from build123d import *

# Parameters (mm, degrees)
SKETCH_W        = 36
SKETCH_H        = 29
SKETCH_R        = 11
PAD_DEPTH       = 7
SKETCH001_R     = 2.5
POCKET_DEPTH    = 29.001
CHAMFER_SIZE    = 1
CHAMFER001_SIZE = 1
CHAMFER002_SIZE = 1


with BuildPart() as part:
    # Sketch → Pad (new body)
    with BuildSketch(Plane.XY):
        Rectangle(SKETCH_W, SKETCH_H)
        Circle(SKETCH_R, mode=Mode.SUBTRACT)
    extrude(amount=PAD_DEPTH)

    # Sketch001 (on Face3 of Pad) → Pocket (cut, through all)
    with BuildSketch(Plane.XZ.offset(14.5)):
        with Locations((13.5, 3.5)):
            Circle(SKETCH001_R)
        with Locations((-13.5, 3.5)):
            Circle(SKETCH001_R)
    extrude(amount=-POCKET_DEPTH, mode=Mode.SUBTRACT)

    # Chamfer
    chamfer_edges = [part.edges().sort_by_distance(p)[0] for p in [
        (18, -14.5, 3.5),
    ]]
    chamfer(chamfer_edges, length=CHAMFER_SIZE)

    # Chamfer001
    chamfer001_edges = [part.edges().sort_by_distance(p)[0] for p in [
        (-18, -14.5, 3.5),
    ]]
    chamfer(chamfer001_edges, length=CHAMFER001_SIZE)

    # Chamfer002
    chamfer002_edges = [part.edges().sort_by_distance(p)[0] for p in [
        (18, 14.5, 3.5),
        (-18, 14.5, 3.5),
    ]]
    chamfer(chamfer002_edges, length=CHAMFER002_SIZE)


solid = part.part
Could you check a few things on this model? Use its own coordinates, in mm. Round coordinates to 2 decimals unless told otherwise and drop trailing zeros. Write each loop counter-clockwise with the first axis right and the second up, starting at its lowest first coordinate (ties: lowest second). Pieces come first, ordered by that corner, then holes. Notation, with made-up numbers: (67.5, 76.5) - (102.5, 76.5) arc R13 ccw to (102.5, 87.5) - close; hole circle Ø2 at (35.25, 32). An arc over 180 degrees is marked (long way). Put each result on its own line as item: value. Start each with the question number.
(1) Thinking about a two-plate mould opening in Z: for faces 1 (the flat face through (-12, 0, 7)), 2 (the cylindrical face through (-16, -0.2, 3.6)), 3 (the flat face through (17.5, 14, 3.5)), 4 (the cylindrical face through (11.66, -0.2, 5.19)), which applies, released by +Z, released by -Z, zero draft, split by the parting line, or undercut?
(2) I want a section at D-D, the plane y = -1.5. Please give me the cut outline in (x, z), plus the area to 3 significant figures.
(3) I want a section at B-B, the plane z = 3.5. Please give me the cut outline in (x, y).
(4) Will this pin go through, and if not, where does the flat tip stop? pin 1 (2 mm diameter, centred on x = 5, y = -11.5, fed in from -Z).
(5) I want a section at A-A, the plane x = 0. Please give me the cut outline in (y, z), plus the area to 3 significant figures.
(6) I need wall thicknesses on probe 1 along X at (y, z) = (6.75, 5); probe 2 along Z at (x, y) = (-13.5, 8.75); probe 3 along X at (y, z) = (-13, 4.5). Which ranges of each line are inside material? Lowest first, please.
(7) I want a section at C-C, the plane y = 12.75. Please give me the cut outline in (x, z).
Here are the results:
1. face 1: released by +Z
1. face 2: undercut
1. face 3: zero draft
1. face 4: undercut
2. outline: (-18, 0) - (-10.9, 0) - (-10.9, 7) - (-18, 7) - close; (10.9, 0) - (18, 0) - (18, 7) - (10.9, 7) - close; hole circle Ø5 at (-13.5, 3.5); hole circle Ø5 at (13.5, 3.5)
2. area: 60.2 mm^2
3. outline: (-18, -13.5) - (-17, -14.5) - (-16, -14.5) - (-16, 14.5) - (-17, 14.5) - (-18, 13.5) - close; (-11, -14.5) - (11, -14.5) - (11, 14.5) - (-11, 14.5) - close; (16, -14.5) - (17, -14.5) - (18, -13.5) - (18, 13.5) - (17, 14.5) - (16, 14.5) - close; hole circle Ø22 at (0, 0)
4. pin 1: stops at z = 0
5. outline: (-14.5, 0) - (-11, 0) - (-11, 7) - (-14.5, 7) - close; (11, 0) - (14.5, 0) - (14.5, 7) - (11, 7) - close
5. area: 49.0 mm^2
6. probe 1: x = -18 to -15.5, -11.5 to -8.69, 8.69 to 11.5, 15.5 to 18
6. probe 2: z = 0 to 1, 6 to 7
6. probe 3: x = -18 to -15.79, -11.21 to 11.21, 15.79 to 18
7. outline: (-18, 0) - (18, 0) - (18, 7) - (-18, 7) - close; hole circle Ø5 at (-13.5, 3.5); hole circle Ø5 at (13.5, 3.5)
